Source: CAD feature listing. Evaluate the final solid. Frame: model axes, mm. A direction names the side the tool comes from. Coordinates: 2 decimals unless noted, no trailing zeros. Write each loop counter-clockwise with the first axis right and the second up, starting at its lowest first coordinate (ties: lowest second). Pieces come first, ordered by that corner, then holes. Notation, with made-up numbers: (53.25, -3.75) - (58.25, -3.75) arc R29 cw to (58.25, 24.25) - close; hole circle Ø9 at (65.25, 88). An arc over 180 degrees is marked (long way). One line per item, written item: value.
from build123d import *

# Parameters (mm, degrees)
SKETCH1_R           = 4
BOSS_EXTRUDE1_DEPTH = 4.5


with BuildPart() as part:
    # Sketch1 → Boss-Extrude1 (new body)
    with BuildSketch(Plane.XY):
        Polygon((152.142010442, -92.754372019), (94.597049202, -63.25), (6.342010442, -108.5), (6.342010442, -147), (46.342010442, -147), align=None)
        with Locations((26.342010442, -140)):
            Circle(SKETCH1_R, mode=Mode.SUBTRACT)
        with Locations((26.342010442, -115.5)):
            Circle(SKETCH1_R, mode=Mode.SUBTRACT)
        Polygon((152.142010442, -33.745627981), (94.597049202, -63.25), (152.142010442, -92.754372019), (209.686971683, -63.25), align=None)
        Polygon((6.342010442, 20.5), (6.342010442, -18), (94.597049202, -63.25), (152.142010442, -33.745627981), (46.342010442, 20.5), align=None)
        with Locations((26.342010442, -11)):
            Circle(SKETCH1_R, mode=Mode.SUBTRACT)
        with Locations((26.342010442, 13.5)):
            Circle(SKETCH1_R, mode=Mode.SUBTRACT)
        Polygon((257.942010442, 20.5), (152.142010442, -33.745627981), (209.686971683, -63.25), (297.942010442, -18), (297.942010442, 20.5), align=None)
        with Locations((277.942010442, -11)):
            Circle(SKETCH1_R, mode=Mode.SUBTRACT)
        with Locations((277.942010442, 13.5)):
            Circle(SKETCH1_R, mode=Mode.SUBTRACT)
        Polygon((209.686971683, -63.25), (152.142010442, -92.754372019), (257.942010442, -147), (297.942010442, -147), (297.942010442, -108.5), align=None)
        with Locations((277.942010442, -140)):
            Circle(SKETCH1_R, mode=Mode.SUBTRACT)
        with Locations((277.942010442, -115.5)):
            Circle(SKETCH1_R, mode=Mode.SUBTRACT)
    extrude(amount=BOSS_EXTRUDE1_DEPTH)


solid = part.part
1) Section query B-B on y = -24.5. Output: boundary loops of the cut face in (x, z), then the cut area to 3 significant figures.
Values found:
outline: (19.02, 0) - (134.11, 0) - (134.11, 4.5) - (19.02, 4.5) - close; (170.17, 0) - (285.26, 0) - (285.26, 4.5) - (170.17, 4.5) - close
area: 1,040 mm2
2) Section query D-D on y = -140. Output: boundary loops of the cut face in (x, z).
Values found:
outline: (6.34, 0) - (22.34, 0) - (22.34, 4.5) - (6.34, 4.5) - close; (30.34, 0) - (59.99, 0) - (59.99, 4.5) - (30.34, 4.5) - close; (244.29, 0) - (273.94, 0) - (273.94, 4.5) - (244.29, 4.5) - close; (281.94, 0) - (297.94, 0) - (297.94, 4.5) - (281.94, 4.5) - close
3) Section query A-A on z = 1.05. State how many separate pieces and enclosed holes the cut face has, then the cut area to 3 significant figures.
Values found:
separate pieces: 1
enclosed holes: 8
area: 29,000 mm2
4) Material intervals for line 1 (X direction, y = 10.5, z = 1.6); line 2 (Y direction, x = 261.5, z = 3.1); line 3 (Y direction, x = 267.5, z = 0.45), sorted ascending.
Values found:
line 1: 6.34 to 23.7, 28.99 to 65.85, 238.44 to 275.3, 280.59 to 297.94
line 2: -147 to -89.82, -36.68 to 20.5
line 3: -147 to -92.89, -33.61 to 20.5
5) Section query C-C on x = 35.5. Output: boundary loops of the cut face in (y, z).
Values found:
outline: (-147, 0) - (-93.55, 0) - (-93.55, 4.5) - (-147, 4.5) - close; (-32.95, 0) - (20.5, 0) - (20.5, 4.5) - (-32.95, 4.5) - close
6) Reachability of faces 1 (the flat face through (99.98, -7, 2.22)), 2 (the flat face through (51.087, -85.558, 2.218)), 3 (the flat face through (99, -120, 2)) from +Z, -Z, +X, -X, +Y, -Y: full face, straight path, thin tool, end or side. Return the list, or none.
Values found:
face 1: +Z, -Z, +Y
face 2: +Z, -Z, -X
face 3: +Z, -Z, -Y
7) Contact query for flat-ended pins moving along their axis: P1, Ø7, axis at x = 26.34, y = -11, coming from the -Z side; P2, Ø1, axis at y = -80, z = 2, coming from the -X side. Output: stop coordinate, or through.
Values found:
P1: through
P2: x = 60.95
8) Draft query along X for faces 4 (the flat face through (254.43, -86.19, 2.22)), 5 (the flat face through (150, -62, 0)), 6 (the cylindrical face through (30.157, 14.701, 2.218)). Return one class per face: released by +X, released by -X, zero draft, split by the parting line, or undercut.
Values found:
face 4: released by +X
face 5: zero draft
face 6: undercut
